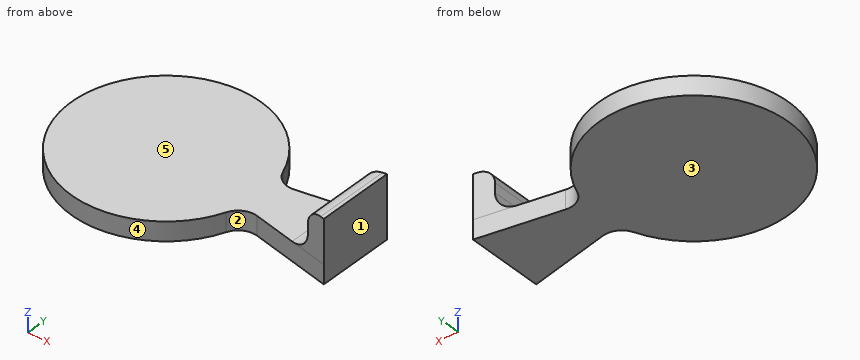
```python
from build123d import *

# Parameters (mm, degrees)
F1_DEPTH = 5
F3_DEPTH = 11.5
F4_R     = 5
F5_R     = 4


with BuildPart() as f1:
    # F0 (on Top) → F1 (new body)
    with BuildSketch(Plane.XY):
        with BuildLine():
            Line((50, 10), (24.494897, 5))
            ThreePointArc((24.494897, 5), (-25, 0), (24.494897, -5))
            Line((24.494897, -5), (50, -10))
            Line((50, -10), (50, 10))
        make_face()
    extrude(amount=F1_DEPTH)

    # F2 (on face) → F3 (join)
    with BuildSketch(Plane.XY.offset(5)):
        Polygon((50, -10), (50, 10), (45, 9.019804), (45, -9.019804), align=None)
    extrude(amount=F3_DEPTH)

    # F4
    f4_edges = [f1.edges().sort_by_distance(p)[0] for p in [
        (24.494897, 5, 2.5),
        (24.494897, -5, 2.5),
        (45, 0, 5),
    ]]
    fillet(f4_edges, radius=F4_R)

    # F5
    f5_edges = [f1.edges().sort_by_distance(p)[0] for p in [
        (45, 0, 16.5),
    ]]
    fillet(f5_edges, radius=F5_R)


solid = f1.part
```
Here's how the part is built. I have some questions about the finished solid (model axes, mm). Face numbers are marked on the shaded views. A direction names the side the tool comes from. Coordinates: 2 decimals unless noted, no trailing zeros. Write each loop counter-clockwise with the first axis right and the second up, starting at its lowest first coordinate (ties: lowest second). Pieces come first, ordered by that corner, then holes. Notation, with made-up numbers: M 40.25,44 L 78.25,44 A18 ccw 78.25,63 Z; hole C 4.5,59.5 d4. An arc over 180 degrees is marked long. Answer as CSV lines item,"result". Start each with the question number.
Q1. Will these pins go through, and if not, where does the flat tip stop? pin 1 Ø1 at (x, y) = (17, 3) entering from +Z; pin 2 Ø2 at (y, z) = (-5.5, 9) entering from -X; pin 3 Ø6 at (x, y) = (27, 14) entering from +Z; pin 4 Ø1.2 at (y, z) = (0, 11) entering from -X.
Q2. If we mould it in two halves opening along X, with no side actions, what happens to the marked faces 1, 2 and 3? For each: pulls with the +X half, pulls with the -X half, needs draft (parallel to the pull), parting line crosses it, or undercut.
Q3. For the marked faces 4 and 5, which set-ups out of +Z, -Z, +X, -X, +Y, -Y let a thin tool reach every point of the face, with its end or its side?
Q4. I need wall thicknesses on probe 1 along Z at (x, y) = (-9, 12.5); probe 2 along X at (y, z) = (23, 3); probe 3 along X at (y, z) = (-5.5, 10.75). Which ranges of each line are inside material? Lowest first, please. Write a range as [from, to].
Q5. Suppose I cut it at C-C, the plane x = 0. List the corners of the cut face in (y, z) for me.
Q6. Suppose I cut it at D-D, the plane x = 13. List the corners of the cut face in (y, z) for me.
Q7. Suppose I cut it at A-A, the plane y = -1. List the corners of the cut face in (x, z) for me.
Q8. Suppose I cut it at B-B, the plane z = 3.75. List the corners of the cut face in (x, y) for me.
Entries:
1,pin 1,"stops at z = 5"
1,pin 2,"stops at x = 44.58"
1,pin 3,"passes through"
1,pin 4,"stops at x = 45"
2,face 1,"pulls with the +X half"
2,face 2,"undercut"
2,face 3,"needs draft"
3,face 4,"+Z, -Z"
3,face 5,"+Z, -X, +Y, -Y"
4,probe 1,"z = [0, 5]"
4,probe 2,"x = [-9.8, 9.8]"
4,probe 3,"x = [45, 50]"
5,outline,"M -25,0 L 25,0 L 25,5 L -25,5 Z"
6,outline,"M -21.35,0 L 21.35,0 L 21.35,5 L -21.35,5 Z"
7,outline,"M -24.98,0 L 50,0 L 50,16.5 L 49,16.5 A4 ccw 45,12.5 L 45,10 A5 cw 40,5 L -24.98,5 Z"
8,outline,"M 23.33,-8.98 A5 cw 28.96,-5.87 L 50,-10 L 50,10 L 28.96,5.87 A5 cw 23.33,8.98 A25 ccw long Z"
